Source: three-view drawing plus pictorial views. Frame: mm from the lowest corner of the part. Give positions to 0.01 mm unless a question says otherwise; leave off trailing zeros. Write each loop counter-clockwise with the first axis right and the second up, starting at its lowest first coordinate (ties: lowest second). Pieces come first, ordered by that corner, then holes. Notation, with made-up numbers: (-1.75, 44.25) -> (24.25, 44.25) arc R15 ccw to (24.25, 62.25) -> close; hole circle Ø7 at (-19.5, 2.5). An arc over 180 degrees is marked (long way). Answer in a Markdown table with one row per item. Add a question column.
Item 1: Draft query along X for the marked faces 1, 2 and 3. Return one class per face: +X half, -X half, draft (parallel to the pull), parting line (faces both ways), or undercut.
Item 2: Section query D-D on y = 10.5. Output: boundary loops of the cut face in (x, z), plus the area to 3 significant figures.
Item 3: Section query C-C on x = 15. Output: boundary loops of the cut face in (y, z).
Item 4: First-contact query: P1, Ø3, axis at x = 16, z = 11, coming from the +Y side; P2, Ø3, axis at x = 20, y = 6, coming from the -Z side; P3, Ø4, axis at y = 12, z = 4, coming from the -X side. Flat tips, straight axial feed; report the tip coordinate or a pass-through.
Item 5: Section query B-B on y = 20.25. Output: boundary loops of the cut face in (x, z), plus the area to 3 significant figures.
Item 6: Section query A-A on z = 15. Output: boundary loops of the cut face in (x, y), plus the area to 3 significant figures.
Item 7: Material intervals for probe 1 along X at (y, z) = (11.5, 15); probe 2 along Y at (x, z) = (23.5, 15); probe 3 along Z at (x, y) = (8, 11.25), sorted ascending. Write a range as from..to.
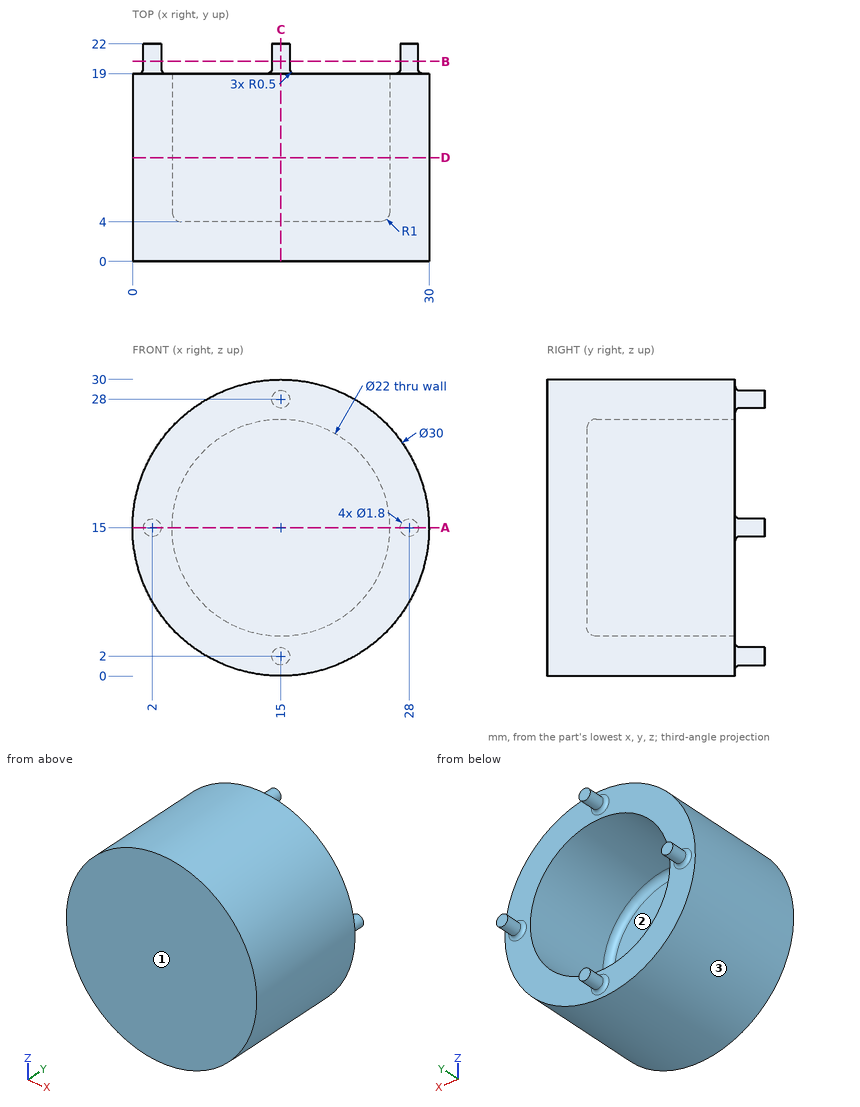
Findings below:
| question | item | result |
|---|---|---|
| 1 | face 1 | draft |
| 1 | face 2 | undercut |
| 1 | face 3 | parting line |
| 2 | outline | circle Ø30 at (15, 15); hole circle Ø22 at (15, 15) |
| 2 | area | 327 mm^2 |
| 3 | outline | (0, 0) -> (19, 0) -> (19, 0.6) arc R0.5 cw to (19.5, 1.1) -> (22, 1.1) -> (22, 2.9) -> (19.5, 2.9) arc R0.5 cw to (19, 3.4) -> (19, 4) -> (5, 4) arc R1 cw to (4, 5) -> (4, 25) arc R1 cw to (5, 26) -> (19, 26) -> (19, 26.6) arc R0.5 cw to (19.5, 27.1) -> (22, 27.1) -> (22, 28.9) -> (19.5, 28.9) arc R0.5 cw to (19, 29.4) -> (19, 30) -> (0, 30) -> close |
| 4 | P1 | stops at y = 4 |
| 4 | P2 | stops at z = 0.41 |
| 4 | P3 | stops at x = 3 |
| 5 | outline | circle Ø1.8 at (2, 15); circle Ø1.8 at (15, 2); circle Ø1.8 at (15, 28); circle Ø1.8 at (28, 15) |
| 5 | area | 10.2 mm^2 |
| 6 | outline | (0, 0) -> (30, 0) -> (30, 19) -> (29.4, 19) arc R0.5 cw to (28.9, 19.5) -> (28.9, 22) -> (27.1, 22) -> (27.1, 19.5) arc R0.5 cw to (26.6, 19) -> (26, 19) -> (26, 5) arc R1 cw to (25, 4) -> (5, 4) arc R1 cw to (4, 5) -> (4, 19) -> (3.4, 19) arc R0.5 cw to (2.9, 19.5) -> (2.9, 22) -> (1.1, 22) -> (1.1, 19.5) arc R0.5 cw to (0.6, 19) -> (0, 19) -> close |
| 6 | area | 251 mm^2 |
| 7 | probe 1 | x = 0..4, 26..30 |
| 7 | probe 2 | y = 0..4 |
| 7 | probe 3 | z = 1.73..6.51, 23.49..28.27 |
